from build123d import *

# Parameters (mm, degrees)
SKETCH1_R           = 22
BOSS_EXTRUDE1_DEPTH = 16
CUT_EXTRUDE1_DEPTH  = 16
BOSS_EXTRUDE2_DEPTH = 12
FILLET1_R           = 2


with BuildPart() as part:
    # Sketch1 → Boss-Extrude1 (new body)
    with BuildSketch(Plane(origin=(0, 0, 0), x_dir=(1, 0, 0), z_dir=(0, 1, 0))):
        with BuildLine():
            Line((37.000000064, 22), (-59, 22))
            Line((-59, 22), (-59, -22))
            Line((-59, -22), (37, -22))
            ThreePointArc((37, -22), (15, 3.2e-08), (37.000000064, 22))
        make_face()
        with Locations((37, 0)):
            Circle(SKETCH1_R)
    extrude(amount=BOSS_EXTRUDE1_DEPTH)

    # Sketch4 → Cut-Extrude1 (cut)
    with BuildSketch(Plane(origin=(0, 16, 0), x_dir=(1, 0, 0), z_dir=(0, 1, 0))):
        with BuildLine():
            Line((37, -8), (13, -8))
            ThreePointArc((13, -8), (5, 0), (13, 8))
            Line((13, 8), (37, 8))
            ThreePointArc((37, 8), (45, 0), (37, -8))
        make_face()
    extrude(amount=-CUT_EXTRUDE1_DEPTH, mode=Mode.SUBTRACT)

    # Sketch5 → Boss-Extrude2 (add)
    with BuildSketch(Plane.XY.offset(22)):
        with BuildLine():
            ThreePointArc((-59, 40), (-51.970562748, 23.029437252), (-35, 16))
            ThreePointArc((-35, 16), (-18.029437252, 23.029437252), (-11, 40))
            Line((-11, 40), (-25, 40))
            ThreePointArc((-25, 40), (-35, 30), (-45, 40))
            Line((-45, 40), (-59, 40))
        make_face()
        with BuildLine():
            ThreePointArc((-11, 40), (-35, 64), (-59, 40))
            Line((-59, 40), (-45, 40))
            ThreePointArc((-45, 40), (-35, 50), (-25, 40))
            Line((-25, 40), (-11, 40))
        make_face()
        with BuildLine():
            Line((-59, 40), (-59, 16))
            Line((-59, 16), (-35, 16))
            ThreePointArc((-35, 16), (-51.970562748, 23.029437252), (-59, 40))
        make_face()
        with BuildLine():
            ThreePointArc((-11, 40), (-18.029437252, 23.029437252), (-35, 16))
            Line((-35, 16), (-11, 16))
            Line((-11, 16), (-11, 40))
        make_face()
    boss_extrude2 = extrude(amount=-BOSS_EXTRUDE2_DEPTH)

    # Mirror1: Boss-Extrude2 across plane
    add(boss_extrude2.mirror(Plane.XY))

    # Fillet1
    fillet1_edges = [part.edges().sort_by_distance(p)[0] for p in [
        (-11, 16, 16),
        (-35, 16, 10),
        (-35, 16, -10),
        (-11, 16, -16),
    ]]
    fillet(fillet1_edges, radius=FILLET1_R)


solid = part.part
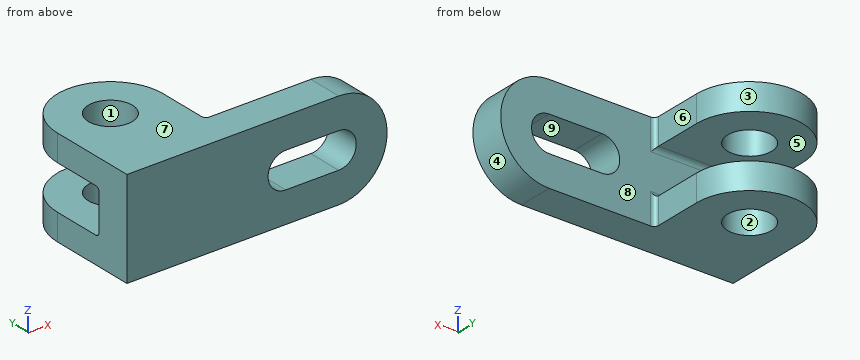
The listing builds one solid part. Answer for the finished solid, in the listing's coordinates (mm). Face numbers are marked on the shaded views. A direction names the side the tool comes from. Give positions to 0.01 mm unless a question says otherwise; leave off trailing zeros. Write each loop counter-clockwise with the first axis right and the second up, starting at its lowest first coordinate (ties: lowest second). Pieces come first, ordered by that corner, then holes. Notation, with made-up numbers: (78.25, 9.5) -> (114.25, 9.5) arc R24 cw to (114.25, 29.5) -> close; hole circle Ø7 at (68.5, 65.25). An arc over 180 degrees is marked (long way). Use a Markdown table: item, result.
(1) Section A-A, the plane z = 0 is taken. Determine the outline of the cut face in (x, y), then the cut area to 3 significant figures.
Return value:
| item | result |
|---|---|
| outline | (-59, 0) -> (5, 0) -> (5, 16) -> (-59, 16) -> close; (45, 0) -> (59, 0) -> (59, 16) -> (45, 16) -> close |
| area | 1,250 mm2 |
(2) Determine the mould class of the marked faces 1, 2, 3 and 4 for opening direction Y: released by +Y, released by -Y, zero draft, split by the parting line, or undercut.
Return value:
| item | result |
|---|---|
| face 1 | undercut |
| face 2 | undercut |
| face 3 | released by +Y |
| face 4 | zero draft |
(3) Find the intervals of material crossed by probe 1 along Y at (x, z) = (-35, -13); probe 2 along Z at (x, y) = (-35, 23); probe 3 along Z at (x, y) = (36.5, 12.5), in increasing order. Write a range as from..to.
Return value:
| item | result |
|---|---|
| probe 1 | 0..30, 50..64 |
| probe 2 | -22..-10, 10..22 |
| probe 3 | -22..-8, 8..22 |
(4) For the marked faces 5, 6, 7, 8 and 9, determine the directions among +Z, -Z, +X, -X, +Y, -Y from which every point of the face is accessible in a straight line to the end or side of a thin tool.
Return value:
| item | result |
|---|---|
| face 5 | +X, -X, +Y |
| face 6 | +Z, -Z, +X, +Y |
| face 7 | +Z, +X, -X, +Y, -Y |
| face 8 | +X, +Y |
| face 9 | +Y, -Y |
(5) Section B-B, the plane y = 23 is taken. Determine the outline of the cut face in (x, z).
Return value:
| item | result |
|---|---|
| outline | (-59, -22) -> (-11, -22) -> (-11, -10) -> (-59, -10) -> close; (-59, 10) -> (-11, 10) -> (-11, 22) -> (-59, 22) -> close |
(6) Section D-D, the plane z = -14 is taken. Determine the outline of the cut face in (x, y).
Return value:
| item | result |
|---|---|
| outline | (-59, 0) -> (53.97, 0) -> (53.97, 16) -> (-9, 16) arc R2 cw to (-11, 18) -> (-11, 40) arc R24 ccw to (-59, 40) -> close; hole circle Ø20 at (-35, 40) |
(7) Flat-ended cylindrical pins translate along their axes: P1, Ø6, axis at y = 51, z = -11, coming from the +X side; P2, Ø3.5, axis at y = 29, z = 13.5, coming from the +X side; P3, Ø6, axis at y = 8.5, z = 17, coming from the +X side; P4, Ø10, axis at y = 55.5, z = 2, coming from the -X side. Find the tip coordinate at first contact, or state that the pin passes through.
Return value:
| item | result |
|---|---|
| P1 | x = -12.37 |
| P2 | x = -11 |
| P3 | x = 53.97 |
| P4 | through |
(8) Section C-C, the plane x = -30 is taken. Determine the outline of the cut face in (y, z), then the cut area to 3 significant figures.
Return value:
| item | result |
|---|---|
| outline | (0, -22) -> (31.34, -22) -> (31.34, -10) -> (18, -10) arc R2 cw to (16, -8) -> (16, 8) arc R2 cw to (18, 10) -> (31.34, 10) -> (31.34, 22) -> (0, 22) -> close; (48.66, -22) -> (63.47, -22) -> (63.47, -10) -> (48.66, -10) -> close; (48.66, 10) -> (63.47, 10) -> (63.47, 22) -> (48.66, 22) -> close |
| area | 1,430 mm2 |
